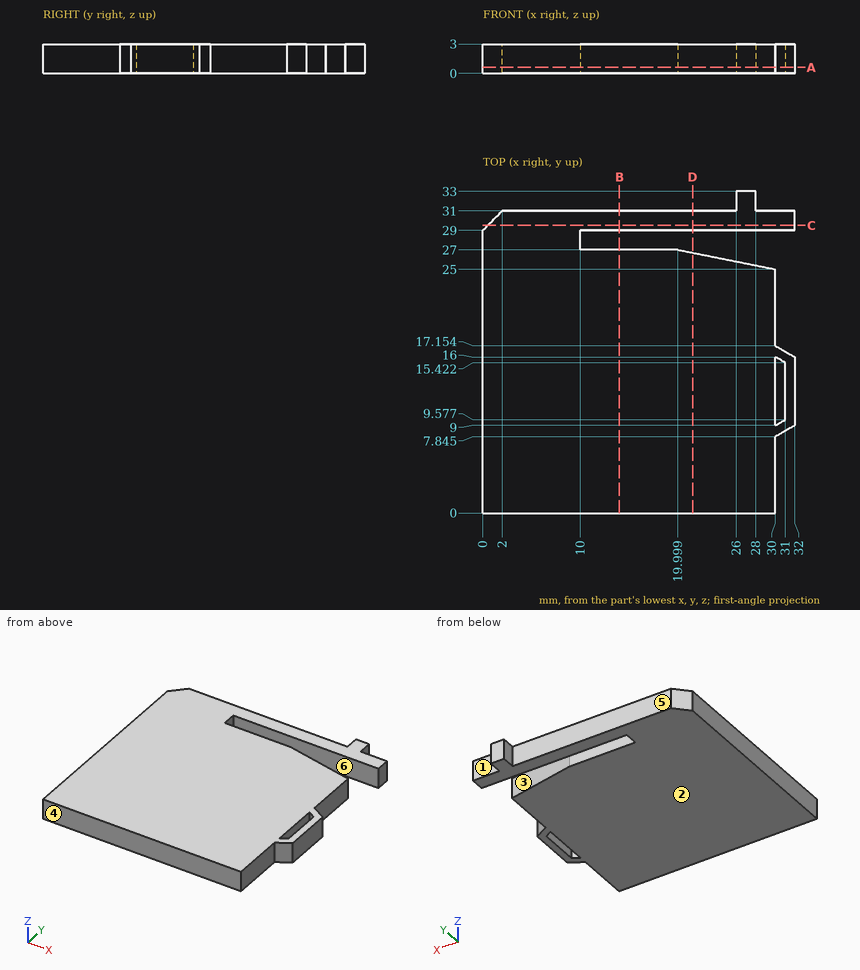
Geometry check sheet. Reference: drawing and pictorial views, mm from the part's lowest x, y, z. A direction names the side the tool comes from. Give positions to 0.01 mm unless a question says otherwise; leave off trailing zeros. Order: outer loops, then holes, each group sorted by start corner. A loop starts at its lowest first (then second) coordinate and runs counter-clockwise, first axis right, second up. Notation, with made-up numbers: M 28.5,41 L 43.5,41 A12 ccw 43.5,46 Z; hole C 42,41 d8. An arc over 180 degrees is marked long. Answer in a Markdown table with one row per item. Add a question column.
Q1. Access from +Z, -Z, +X, -X, +Y, -Y to the whole of each face (thin tool, end or side, straight path). Record for the marked faces 1 and 2.
Q2. Gauge pin test, flat ends, axial feed: pin 1 Ø4 at (x, y) = (17.5, 23.5) entering from -Z; pin 2 Ø0.9 at (x, z) = (15.5, 1) entering from +Y; pin 3 Ø0.9 at (y, z) = (19.5, 1.5) entering from +X; pin 4 Ø0.6 at (y, z) = (31.5, 2) entering from +X. Record the tip position at first contact, or that the pin passes through.
Q3. Sectioned sample at C-C, the plane y = 29.5. Record the boundary of the cut face in (x, z).
Q4. Sectioned sample at A-A, the plane z = 0.6. Record the boundary of the cut face in (x, y) (1 decimal), and give its area (3 significant figures).
Q5. Sectioned sample at B-B, the plane x = 14. Record the boundary of the cut face in (y, z).
Q6. Release check for a two-part mould opening along Y. For the marked faces 3, 4, 5 and 6 record: released by +Y, released by -Y, zero draft, split by the parting line, or undercut.
Q7. Thickness scan on L1, parallel to Y at x = 20, z = 2.9; L2, parallel to X at y = 15, z = 0.6; L3, parallel to X at y = 32, z = 0.4. Record the ranges inside material, lowest first.
Q8. Sectioned sample at D-D, the plane x = 21.5. Record the boundary of the cut face in (y, z).
Verdict:
| question | item | result |
|---|---|---|
| 1 | face 1 | +Z, -Z, +X, +Y |
| 1 | face 2 | -Z, +X, -X, +Y, -Y |
| 2 | pin 1 | z = 0 |
| 2 | pin 2 | y = 31 |
| 2 | pin 3 | x = 30 |
| 2 | pin 4 | x = 28 |
| 3 | outline | M 0.5,0 L 32,0 L 32,3 L 0.5,3 Z |
| 4 | outline | M 0,0 L 30,0 L 30,7.8 L 32,9 L 32,16 L 30,17.2 L 30,25 L 20,27 L 10,27 L 10,29 L 32,29 L 32,31 L 28,31 L 28,33 L 26,33 L 26,31 L 2,31 L 0,29 Z; hole M 30,9 L 31,9.6 L 31,15.4 L 30,16 Z |
| 4 | area | 896 mm² |
| 5 | outline | M 0,0 L 27,0 L 27,3 L 0,3 Z; M 29,0 L 31,0 L 31,3 L 29,3 Z |
| 6 | face 3 | undercut |
| 6 | face 4 | released by -Y |
| 6 | face 5 | released by +Y |
| 6 | face 6 | undercut |
| 7 | L1 | 0 to 27, 29 to 31 |
| 7 | L2 | 0 to 30, 31 to 32 |
| 7 | L3 | 26 to 28 |
| 8 | outline | M 0,0 L 26.7,0 L 26.7,3 L 0,3 Z; M 29,0 L 31,0 L 31,3 L 29,3 Z |
